Design review of the part built by this model. Coordinates are the model's own, in mm. Face numbers are marked on the shaded views. Coordinates: 2 decimals unless noted, no trailing zeros. Loops run counter-clockwise (first coordinate to the right, second up) from the corner with the lowest first, then second, coordinate; pieces in that order, holes last. Notation, with made-up numbers: (88, -18) -> (122, -18) arc R16 ccw to (122, -3) -> close; hole circle Ø7 at (39.25, 66). An arc over 180 degrees is marked (long way). Answer in a Markdown table with one row per item.
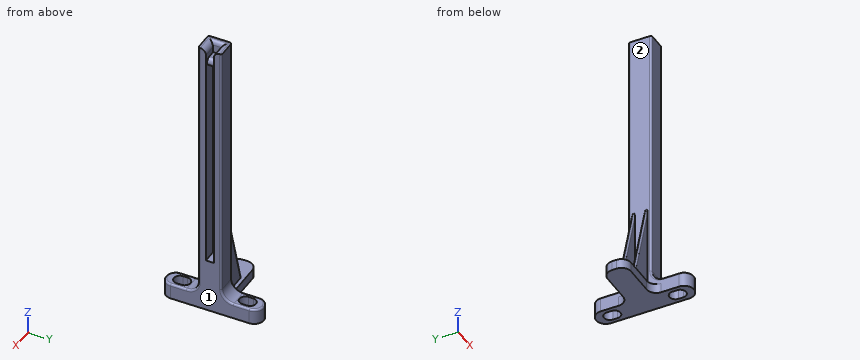
```python
from build123d import *

# Parameters (mm, degrees)
SKETCH_W        = 10
SKETCH_H        = 50
PAD_DEPTH       = 8
SKETCH001_W     = 10
SKETCH001_H     = 12
PAD001_DEPTH    = 140
SKETCH002_W     = 4
SKETCH002_H     = 120
POCKET_DEPTH    = 7
POCKET001_DEPTH = 8.001
SKETCH004_W     = 12
SKETCH004_H     = 5
PAD002_DEPTH    = 25
SKETCH005_W     = 1.5
SKETCH005_H     = 45
PAD003_DEPTH    = 13
POCKET002_DEPTH = 29.001
FILLET_R        = 4.9
FILLET001_R     = 6
FILLET002_R     = 0.7
FILLET003_R     = 1
SKETCH007_W     = 4
SKETCH007_H     = 3
PAD004_DEPTH    = 6
FILLET004_R     = 2.3
FILLET005_R     = 3
FILLET006_R     = 2


with BuildPart() as part:
    # Sketch → Pad (new body)
    with BuildSketch(Plane.XY):
        with Locations((-17.676624, 11.727997)):
            Rectangle(SKETCH_W, SKETCH_H)
    extrude(amount=PAD_DEPTH)

    # Sketch001 (on Face6 of Pad) → Pad001 (join)
    with BuildSketch(Plane.XY.offset(8)):
        with Locations((-17.676624, 11.727997)):
            Rectangle(SKETCH001_W, SKETCH001_H)
    extrude(amount=PAD001_DEPTH)

    # Sketch002 (on Face9 of Pad001) → Pocket (cut)
    with BuildSketch(Plane.YZ.offset(-12.676624)):
        with Locations((11.727997, 88)):
            Rectangle(SKETCH002_W, SKETCH002_H)
    extrude(amount=-POCKET_DEPTH, mode=Mode.SUBTRACT)

    # Sketch003 (on Face7 of Pocket) → Pocket001 (cut, through all)
    with BuildSketch(Plane.XY.offset(8)):
        with BuildLine():
            ThreePointArc((-14.676624, -3.772003), (-17.676624, -0.772003), (-20.676624, -3.772003))
            Line((-20.676624, -3.772003), (-20.676624, -6.272003))
            ThreePointArc((-20.676624, -6.272003), (-17.676624, -9.272003), (-14.676624, -6.272003))
            Line((-14.676624, -3.772003), (-14.676624, -6.272003))
        make_face()
        with BuildLine():
            ThreePointArc((-14.676624, 29.727997), (-17.676624, 32.727997), (-20.676624, 29.727997))
            Line((-20.676624, 29.727997), (-20.676624, 27.227997))
            ThreePointArc((-20.676624, 27.227997), (-17.676624, 24.227997), (-14.676624, 27.227997))
            Line((-14.676624, 29.727997), (-14.676624, 27.227997))
        make_face()
    extrude(amount=-POCKET001_DEPTH, mode=Mode.SUBTRACT)

    # Sketch004 (on Face2 of Pocket001) → Pad002 (join)
    with BuildSketch(Plane(origin=(-22.676624, 0, 0), x_dir=(0, -1, 0), z_dir=(-1, 0, 0))):
        with Locations((-11.727997, 2.5)):
            Rectangle(SKETCH004_W, SKETCH004_H)
    extrude(amount=PAD002_DEPTH)

    # Sketch005 (on Face9 of Pad002) → Pad003 (join)
    with BuildSketch(Plane(origin=(-22.676624, 0, 0), x_dir=(0, -1, 0), z_dir=(-1, 0, 0))):
        with Locations((-8.477997, 27.5)):
            Rectangle(SKETCH005_W, SKETCH005_H)
        with Locations((-14.977997, 27.5)):
            Rectangle(SKETCH005_W, SKETCH005_H)
    extrude(amount=PAD003_DEPTH)

    # Sketch006 (on Face29 of Pad003) → Pocket002 (cut, through all)
    with BuildSketch(Plane.XZ.offset(-7.727997)):
        Polygon((-35.676624, 5), (-22.676624, 50), (-35.676624, 50), align=None)
    extrude(amount=-POCKET002_DEPTH, mode=Mode.SUBTRACT)

    # Fillet
    fillet_edges = [part.edges().sort_by_distance(p)[0] for p in [
        (-12.676624, 36.727997, 4),
        (-22.676624, 36.727997, 4),
        (-22.676624, 17.727997, 2.5),
        (-47.676624, 17.727997, 2.5),
        (-47.676624, 5.727997, 2.5),
        (-22.676624, 5.727997, 2.5),
        (-22.676624, -13.272003, 4),
        (-12.676624, -13.272003, 4),
    ]]
    fillet(fillet_edges, radius=FILLET_R)

    # Fillet001
    fillet001_edges = [part.edges().sort_by_distance(p)[0] for p in [
        (-17.676624, 5.727997, 8),
        (-17.676624, 17.727997, 8),
    ]]
    fillet(fillet001_edges, radius=FILLET001_R)

    # Fillet002
    fillet002_edges = [part.edges().sort_by_distance(p)[0] for p in [
        (-29.176624, 7.727997, 27.5),
        (-29.176624, 9.227997, 27.5),
        (-29.176624, 14.227997, 27.5),
        (-29.176624, 15.727997, 27.5),
    ]]
    fillet(fillet002_edges, radius=FILLET002_R)

    # Fillet003
    fillet003_edges = [part.edges().sort_by_distance(p)[0] for p in [
        (-22.676624, 5.727997, 81),
        (-22.676624, 17.727997, 99),
    ]]
    fillet(fillet003_edges, radius=FILLET003_R)

    # Sketch007 (on Face57 of Fillet003) → Pad004 (join)
    with BuildSketch(Plane.YZ.offset(-19.676624)):
        with Locations((11.727997, 140.5)):
            Rectangle(SKETCH007_W, SKETCH007_H)
    extrude(amount=PAD004_DEPTH)

    # Fillet004
    fillet004_edges = [part.edges().sort_by_distance(p)[0] for p in [
        (-13.676624, 11.727997, 142),
    ]]
    fillet(fillet004_edges, radius=FILLET004_R)

    # Fillet005
    fillet005_edges = [part.edges().sort_by_distance(p)[0] for p in [
        (-16.176624, 9.727997, 148),
        (-16.176624, 13.727997, 148),
    ]]
    fillet(fillet005_edges, radius=FILLET005_R)

    # Fillet006
    fillet006_edges = [part.edges().sort_by_distance(p)[0] for p in [
        (-19.676624, 11.727997, 148),
    ]]
    fillet(fillet006_edges, radius=FILLET006_R)


solid = part.part
```
(1) For pin 1 (6.5 mm diameter, centred on x = -16, z = 55.5, fed in from -Y); pin 2 (10 mm diameter, centred on x = -16.5, y = 10.5, fed in from +Z); pin 3 (4 mm diameter, centred on x = -19.5, y = -7, fed in from +Z); pin 4 (3.5 mm diameter, centred on x = -30, z = 19.5, fed in from +Y), all flat-tipped, find the tip position at first contact; note any pin that passes through.
Evaluation:
| item | result |
|---|---|
| pin 1 | stops at y = 5.73 |
| pin 2 | stops at z = 148 |
| pin 3 | stops at z = 8 |
| pin 4 | stops at y = 15.73 |
(2) To check wall thickness, follow probe 1 along Y at (x, z) = (-17, 50.5); probe 2 along Z at (x, y) = (-13.5, 26.5); probe 3 along X at (y, z) = (13.5, 80.5). State the ranges of each line that lie inside material, in increasing order.
Evaluation:
| item | result |
|---|---|
| probe 1 | y = 5.73 to 9.73, 13.73 to 17.73 |
| probe 2 | z = 0 to 7.98 |
| probe 3 | x = -22.68 to -19.68 |
(3) Take a section at B-B on x = -41. Give the boundary of the cut face in (y, z), and give its area (3 significant figures).
Evaluation:
| item | result |
|---|---|
| outline | (5.73, 0) -> (17.73, 0) -> (17.73, 5) -> (5.73, 5) -> close |
| area | 60.0 mm² |
(4) Take a section at A-A on z = 130.5. Give the boundary of the cut face in (x, y), and give its area (3 significant figures).
Evaluation:
| item | result |
|---|---|
| outline | (-22.68, 6.73) arc R1 ccw to (-21.68, 5.73) -> (-13.68, 5.73) arc R1 ccw to (-12.68, 6.73) -> (-12.68, 9.73) -> (-19.68, 9.73) -> (-19.68, 13.73) -> (-12.68, 13.73) -> (-12.68, 16.73) arc R1 ccw to (-13.68, 17.73) -> (-21.68, 17.73) arc R1 ccw to (-22.68, 16.73) -> close |
| area | 91.1 mm² |
(5) Draft analysis for pull direction Y (two halves, no side actions). For the marked faces 1 and 2, state which applies: pulls with the +Y half, pulls with the -Y half, needs draft (parallel to the pull), parting line crosses it, or undercut.
Evaluation:
| item | result |
|---|---|
| face 1 | needs draft |
| face 2 | undercut |
